For this review, take the finished solid that the model builds, in its own axes (mm). Face numbers are marked on the shaded views. A direction names the side the tool comes from. Give positions to 0.01 mm unless a question says otherwise; leave off trailing zeros. Order: outer loops, then holes, each group sorted by start corner. A loop starts at its lowest first (then second) coordinate and runs counter-clockwise, first axis right, second up. Notation, with made-up numbers: (19, -30) - (66, -30) arc R20 cw to (66, -13) - close; hole circle Ø11 at (18, -30.75). An arc over 180 degrees is marked (long way). Use a Markdown table: item, result. Add a question column.
1) Clearance check with flat-ended pins moving along their axes: P1, Ø14.5, axis at x = 12.7, y = -12.7, coming from the +Z side; P2, Ø7.5, axis at y = -17.5, z = 35, coming from the -X side; P3, Ø2, axis at y = -20.5, z = 13.5, coming from the +X side. State where each tip first meets the part, or that it passes through.
2) Mouldability with a two-part tool opening along Y and no side actions: class the marked faces 1, 2, 3 and 4 as released by +Y, released by -Y, zero draft, split by the parting line, or undercut.
3) We need section C-C on z = 23.5. Write out the cut boundary in (x, y), then the cut area to 3 significant figures.
4) We need section A-A on y = -8.25. Write out the cut boundary in (x, z), then the cut area to 3 significant figures.
5) We need section D-D on z = 9. Write out the cut boundary in (x, y).
6) Machinability: for the marked faces 5, 6 and 7, which of the approach directions +Z, -Z, +X, -X, +Y, -Y give a long, thin tool a straight path to every point of the face, cutting with its end or side? Answer none if there is none.
7) Wall thickness on L1, parallel to Y at x = 63.5, z = 3.25; L2, parallel to Z at x = 22, y = -15; L3, parallel to Z at x = 44.5, y = -12.7 (3 decimals): over which ranges is each line inside the solid? List them lowest first.
8) We need section B-B on x = 60. Write out the cut boundary in (y, z).
```python
from build123d import *

# Parameters (mm, degrees)
F0_W     = 76.2
F0_H     = 44.45
F1_DEPTH = 25.4
F2_W     = 25.4
F2_H     = 31.75
F3_DEPTH = 25.4
F4_R     = 6.35
F5_DEPTH = 25.4
F6_R     = 6.35
F7_DEPTH = 25.4
F8_R     = 6.35
F9_DEPTH = 25.4


with BuildPart() as f1:
    # F0 (on Front) → F1 (new body)
    with BuildSketch(Plane.XZ):
        with Locations((38.1, 22.225)):
            Rectangle(F0_W, F0_H)
    extrude(amount=F1_DEPTH)

    # F2 (on face) → F3 (cut)
    with BuildSketch(Plane.XZ.offset(25.4)):
        with Locations((12.7, 28.575)):
            Rectangle(F2_W, F2_H)
        with Locations((63.5, 28.575)):
            Rectangle(F2_W, F2_H)
    extrude(amount=-F3_DEPTH, mode=Mode.SUBTRACT)

    # F4 (on face) → F5 (cut)
    with BuildSketch(Plane.YZ.offset(50.8)):
        with Locations((-12.7, 28.575)):
            Circle(F4_R)
        with BuildLine():
            ThreePointArc((-12.7000002087, 44.45), (-4.5680322999, 41.5974597921), (0, 34.29))
            Line((0, 34.29), (0, 44.45))
            Line((0, 44.45), (-12.7000002087, 44.45))
        make_face()
        with BuildLine():
            ThreePointArc((-25.4, 34.29), (-20.831967863, 41.5974596617), (-12.7000002087, 44.45))
            Line((-12.7000002087, 44.45), (-25.4, 44.45))
            Line((-25.4, 44.45), (-25.4, 34.29))
        make_face()
    extrude(amount=-F5_DEPTH, mode=Mode.SUBTRACT)

    # F6 (on face) → F7 (cut)
    with BuildSketch(Plane.XY.offset(12.7)):
        with Locations((63.5, -12.7)):
            Circle(F6_R)
        with BuildLine():
            ThreePointArc((63.5, 0), (72.4802561211, -3.7197438789), (76.2, -12.7))
            Line((76.2, -12.7), (76.2, 0))
            Line((76.2, 0), (63.5, 0))
        make_face()
        with BuildLine():
            ThreePointArc((76.2, -12.7), (72.4802561211, -21.6802561211), (63.5, -25.4))
            Line((63.5, -25.4), (76.2, -25.4))
            Line((76.2, -25.4), (76.2, -12.7))
        make_face()
    extrude(amount=-F7_DEPTH, mode=Mode.SUBTRACT)

    # F8 (on face) → F9 (cut)
    with BuildSketch(Plane.XY.offset(12.7)):
        with BuildLine():
            ThreePointArc((0, -12.7), (3.7197438789, -3.7197438789), (12.7, 0))
            Line((12.7, 0), (0, 0))
            Line((0, 0), (0, -12.7))
        make_face()
        with Locations((12.7, -12.7)):
            Circle(F8_R)
        with BuildLine():
            ThreePointArc((12.7, -25.4), (3.7197438789, -21.6802561211), (0, -12.7))
            Line((0, -12.7), (0, -25.4))
            Line((0, -25.4), (12.7, -25.4))
        make_face()
    extrude(amount=-F9_DEPTH, mode=Mode.SUBTRACT)


solid = f1.part
```
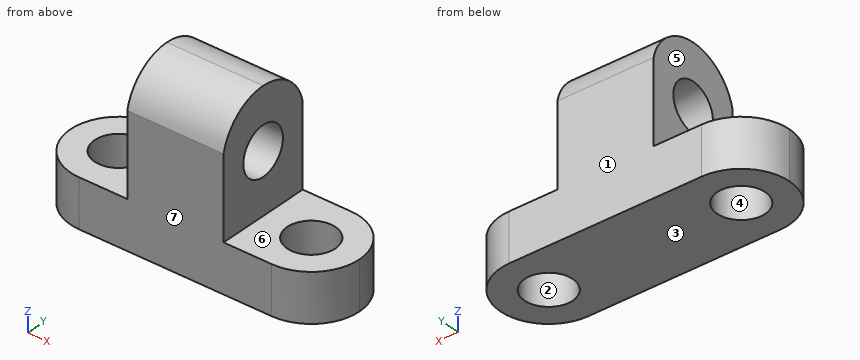
Checked values:
| question | item | result |
|---|---|---|
| 1 | P1 | z = 12.7 |
| 1 | P2 | x = 25.4 |
| 1 | P3 | x = 73.96 |
| 2 | face 1 | released by +Y |
| 2 | face 2 | undercut |
| 2 | face 3 | zero draft |
| 2 | face 4 | undercut |
| 3 | outline | (25.4, -25.4) - (50.8, -25.4) - (50.8, -16.52) - (25.4, -16.52) - close; (25.4, -8.88) - (50.8, -8.88) - (50.8, 0) - (25.4, 0) - close |
| 3 | area | 451 mm² |
| 4 | outline | (0.81, 0) - (8.17, 0) - (8.17, 12.7) - (0.81, 12.7) - close; (17.23, 0) - (58.97, 0) - (58.97, 12.7) - (50.8, 12.7) - (50.8, 24.05) - (25.4, 24.05) - (25.4, 12.7) - (17.23, 12.7) - close; (25.4, 33.1) - (50.8, 33.1) - (50.8, 43.67) - (25.4, 43.67) - close; (68.03, 0) - (75.39, 0) - (75.39, 12.7) - (68.03, 12.7) - close |
| 4 | area | 1,270 mm² |
| 5 | outline | (12.7, -25.4) - (63.5, -25.4) arc R12.7 ccw to (63.5, 0) - (12.7, 0) arc R12.7 ccw to start; hole circle Ø12.7 at (12.7, -12.7); hole circle Ø12.7 at (63.5, -12.7) |
| 6 | face 5 | +Z, -X, +Y, -Y |
| 6 | face 6 | +Z, +X, +Y, -Y |
| 6 | face 7 | +Z, -Z, +X, -X, -Y |
| 7 | L1 | -25.4 to -19.05, -6.35 to 0 |
| 7 | L2 | 0 to 12.7 |
| 7 | L3 | 0 to 22.225, 34.925 to 44.45 |
| 8 | outline | (-25.4, 0) - (-18, 0) - (-18, 12.7) - (-25.4, 12.7) - close; (-7.4, 0) - (0, 0) - (0, 12.7) - (-7.4, 12.7) - close |
